Source: CAD feature listing. Evaluate the final solid. Frame: model axes, mm. Face numbers are marked on the shaded views. A direction names the side the tool comes from. Coordinates: 2 decimals unless noted, no trailing zeros. Write each loop counter-clockwise with the first axis right and the second up, starting at its lowest first coordinate (ties: lowest second). Pieces come first, ordered by that corner, then holes. Notation, with made-up numbers: M -1,-21 L 28,-21 A24 cw 28,-4 Z; hole C 18,12 d6. An arc over 180 degrees is marked long. One line per item, written item: value. Start each with the question number.
Item 1: Cut plane A-A, the plane x = 15. Output: boundary loops of the cut face in (y, z), then the cut area to 3 significant figures.
Item 2: Mould query, pull axis X, two halves, no side actions, for the marked faces 1, 2, 3 and 4. Classes: released by +X, released by -X, zero draft, split by the parting line, or undercut.
Item 3: Ray query, L1, parallel to X at y = -22.5, z = -10; L2, parallel to Y at x = 10, z = -2.75; L3, parallel to Z at x = 23, y = -22.5. Return the intervals inside material, ascending. Write a range as from..to.
Item 4: Cut plane C-C, the plane x = -6. Output: boundary loops of the cut face in (y, z).
Item 5: Set-up query: the marked faces 5, 6, 7 and 8. Return all of +Z, -Z, +X, -X, +Y, -Y with unobstructed straight access to the full face (end or side cutting, diameter ignored); none if empty.
Item 6: Cut plane D-D, the plane y = -11. Output: boundary loops of the cut face in (x, z), then the cut area to 3 significant figures.
Item 7: Cut plane B-B, the plane z = -4. State how many separate pieces and enclosed holes the cut face has, then the cut area to 3 significant figures.
Item 8: Pin query (flat end, axial travel): P1, Ø10, axis at x = 3.5, y = 0, coming from the -Z side; P2, Ø4, axis at y = 8.5, z = -3, coming from the -X side; P3, Ø1.5, axis at x = -9, z = -5.5, coming from the -Y side; P4, Ø6, axis at y = -22.5, z = -3.5, coming from the +X side. Return the tip coordinate at first contact, or that it passes through.
```python
from build123d import *

# Parameters (mm, degrees)
BOSS_EXTRUDE1_DEPTH = 2
BOSS_EXTRUDE2_DEPTH = 16
SKETCH2_R           = 2
SKETCH2_R_2         = 1
BOSS_EXTRUDE3_DEPTH = 8
SKETCH3_R           = 8
CUT_EXTRUDE1_DEPTH  = 8
SKETCH4_W           = 15.5
SKETCH4_H           = 6.9
SKETCH4_W_2         = 13
SKETCH4_H_2         = 4
BOSS_EXTRUDE4_DEPTH = 8
SKETCH4_2_W         = 13
SKETCH4_2_H         = 4
SKETCH4_2_R         = 4
CUT_EXTRUDE2_DEPTH  = 8


with BuildPart() as part:
    # Sketch1 → Boss-Extrude1 (new body)
    with BuildSketch(Plane.XY):
        with BuildLine():
            Line((-43.5, 19), (43.5, 19))
            ThreePointArc((43.5, 19), (62.5, 0), (43.5, -19))
            Line((43.5, -19), (-43.5, -19))
            ThreePointArc((-43.5, -19), (-62.5, 0), (-43.5, 19))
        make_face()
    extrude(amount=BOSS_EXTRUDE1_DEPTH)

    # Sketch1_3 → Boss-Extrude2 (add)
    with BuildSketch(Plane.XY):
        with BuildLine():
            Line((-43.5, 19), (43.5, 19))
            ThreePointArc((43.5, 19), (62.5, 0), (43.5, -19))
            Line((43.5, -19), (-43.5, -19))
            ThreePointArc((-43.5, -19), (-62.5, 0), (-43.5, 19))
        make_face()
        with BuildLine():
            Line((-43.5, 17), (43.5, 17))
            ThreePointArc((43.5, 17), (60.5, 0), (43.5, -17))
            Line((43.5, -17), (-43.5, -17))
            ThreePointArc((-43.5, -17), (-60.5, 0), (-43.5, 17))
        make_face(mode=Mode.SUBTRACT)
    extrude(amount=-BOSS_EXTRUDE2_DEPTH)

    # Sketch2 → Boss-Extrude3 (add)
    with BuildSketch(Plane(origin=(0, 0, 0), x_dir=(-1, 0, 0), z_dir=(0, 0, -1))):
        with Locations((-40, 15.1)):
            Circle(SKETCH2_R)
        with Locations((-40, 15.1)):
            Circle(SKETCH2_R_2, mode=Mode.SUBTRACT)
        with Locations((-10, 15.1)):
            Circle(SKETCH2_R)
        with Locations((-10, 15.1)):
            Circle(SKETCH2_R_2, mode=Mode.SUBTRACT)
        with Locations((-40, 0.1)):
            Circle(SKETCH2_R)
        with Locations((-40, 0.1)):
            Circle(SKETCH2_R_2, mode=Mode.SUBTRACT)
        with Locations((-10, 0.1)):
            Circle(SKETCH2_R)
        with Locations((-10, 0.1)):
            Circle(SKETCH2_R_2, mode=Mode.SUBTRACT)
        with Locations((10, 15.1)):
            Circle(SKETCH2_R)
        with Locations((10, 15.1)):
            Circle(SKETCH2_R_2, mode=Mode.SUBTRACT)
        with Locations((40, 15.1)):
            Circle(SKETCH2_R)
        with Locations((40, 15.1)):
            Circle(SKETCH2_R_2, mode=Mode.SUBTRACT)
        with Locations((10, 0.1)):
            Circle(SKETCH2_R)
        with Locations((10, 0.1)):
            Circle(SKETCH2_R_2, mode=Mode.SUBTRACT)
        with Locations((40, 0.1)):
            Circle(SKETCH2_R)
        with Locations((40, 0.1)):
            Circle(SKETCH2_R_2, mode=Mode.SUBTRACT)
    extrude(amount=BOSS_EXTRUDE3_DEPTH)

    # Sketch3 → Cut-Extrude1 (cut)
    with BuildSketch(Plane(origin=(0, 0, 0), x_dir=(-1, 0, 0), z_dir=(0, 0, -1))):
        with Locations((30, 8.1)):
            Circle(SKETCH3_R)
        with Locations((-30, 8.1)):
            Circle(SKETCH3_R)
    extrude(amount=-CUT_EXTRUDE1_DEPTH, mode=Mode.SUBTRACT)

    # Sketch4 → Boss-Extrude4 (add)
    with BuildSketch(Plane.XZ.offset(19)):
        with Locations((-19.25, -11.45)):
            Rectangle(SKETCH4_W, SKETCH4_H)
        with Locations((-19.25, -11.45)):
            Rectangle(SKETCH4_W_2, SKETCH4_H_2, mode=Mode.SUBTRACT)
        with Locations((19.25, -11.45)):
            Rectangle(SKETCH4_W, SKETCH4_H)
        with Locations((19.25, -11.45)):
            Rectangle(SKETCH4_W_2, SKETCH4_H_2, mode=Mode.SUBTRACT)
    extrude(amount=BOSS_EXTRUDE4_DEPTH)

    # Sketch4_2 → Cut-Extrude2 (cut)
    with BuildSketch(Plane.XZ.offset(19)):
        with Locations((19.25, -11.45)):
            Rectangle(SKETCH4_2_W, SKETCH4_2_H)
        with Locations((-19.25, -11.45)):
            Rectangle(SKETCH4_2_W, SKETCH4_2_H)
        with Locations((0, -11.45)):
            Circle(SKETCH4_2_R)
    extrude(amount=-CUT_EXTRUDE2_DEPTH, mode=Mode.SUBTRACT)


solid = part.part
```
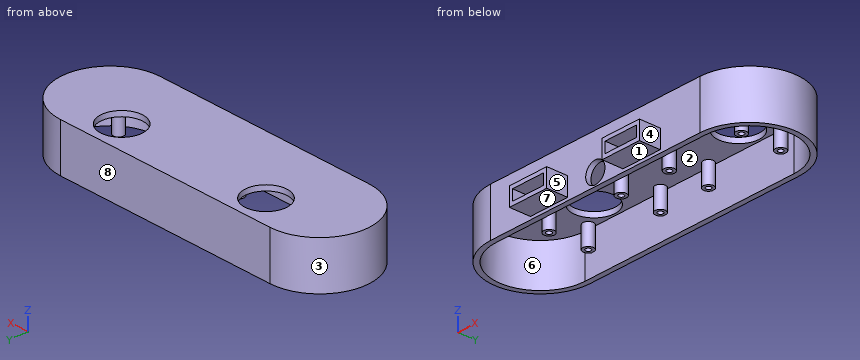
From the geometry:
1. outline: M -27,-14.9 L -19,-14.9 L -19,-16 L -17,-16 L -17,-13.45 L -27,-13.45 Z; M -27,-9.45 L -17,-9.45 L -17,0 L 17,0 L 17,-16 L 19,-16 L 19,2 L -19,2 L -19,-8 L -27,-8 Z
1. area: 155 mm²
2. face 1: zero draft
2. face 2: undercut
2. face 3: released by -X
2. face 4: released by +X
3. L1: x = -27..-25.75, -12.75..-11.5, 11.5..12.75, 25.75..27
3. L2: y = -19..-17, -1.9..-0.9, 1.1..2.1, 13.1..14.1, 16.1..19
3. L3: z = -14.9..-13.45, -9.45..-8
4. outline: M -19,-16 L -17,-16 L -17,0 L 17,0 L 17,-16 L 19,-16 L 19,2 L -19,2 Z
5. face 5: +Z, -Z, -Y
5. face 6: -Z
5. face 7: -Z, +X, -X, -Y
5. face 8: +Z, -Z, +X, -X, +Y
6. outline: M -58.99,-16 L -56.46,-16 L -56.46,0 L 56.46,0 L 56.46,-16 L 58.99,-16 L 58.99,2 L -58.99,2 Z
6. area: 317 mm²
7. separate pieces: 5
7. enclosed holes: 9
7. area: 649 mm²
8. P1: stops at z = -8
8. P2: stops at x = -61.35
8. P3: stops at y = -19
8. P4: passes through
